For this review, take the finished solid that the model builds, in its own axes (mm). Round coordinates to 2 decimals unless told otherwise and drop trailing zeros. Loops run counter-clockwise (first coordinate to the right, second up) from the corner with the lowest first, then second, coordinate; pieces in that order, holes last.
1. Clearance check with flat-ended pins moving along their axes: pin 1 Ø10 at (x, y) = (-1.5, 80.5) entering from -Z; pin 2 Ø5.5 at (x, z) = (53.34, -76.18) entering from -Y; pin 3 Ø6.5 at (x, z) = (-92, 17) entering from -Y; pin 4 Ø8 at (y, z) = (87.5, 65.5) entering from -X. State where each tip first meets the part, or that it passes through.
2. To check wall thickness, follow line 1 along Z through (x, y) = (-49.5, 16); line 2 along Z through (x, y) = (29, 10); line 3 along Z through (x, y) = (0, 11). State the ranges of each line that lie inside material, in increasing order.
3. Draft analysis for pull direction Z (two halves, no side actions). For faces 1 (the flat face through (92, 13.7, -16)), 2 (the flat face through (-1, 0, -1)), 3 (the flat face through (86.75, 5.18, -33.3)), state which applies: released by +Z, released by -Z, zero draft, split by the parting line, or undercut.
4. Consider section A-A on x = 0. State the section outline as (y, z) points, then the cut area to 3 significant figures.
5. Consider section D-D on y = 52. State the section outline as (x, z) points.
6. Consider section B-B on y = 8. State the section outline as (x, z) points.
7. Consider section C-C on z = 44.5. State the section outline as (x, y) points.
Autodesk Fusion 360 part; units mm, degrees
sketch "Sketch1" plane through (0, 0, 0) normal (0, 0, 1) x (1, 0, 0)
  line L0 (0, 0) -> (102, 0)
  line L1 (0, 0) -> (0, 102)
  arc A0 (102, 0) -> (0, 102) centre (0, 0) ccw
  dimension "d1" = 204
revolve "Revolve1" add sketch "Sketch1" angle 360 about axis through (0, 0, 0) along (0, 1, 0)
sketch "Sketch2" plane through (0, 0, 0) normal (0, -1, 0) x (1, 0, 0)
  circle A0 centre (0, 0) radius 102
  line L0 (0, 0) -> (0, -0.5) construction
  line L1 (0, -0.5) -> (-40.4969, -0.5) construction
  line L2 (-40.4969, -0.5) -> (40.4969, -0.5)
  arc A1 (40.4969, -0.5) -> (-40.4969, -0.5) centre (0, 0) ccw
  dimension "d3" = 81
  dimension "d4" = 0.5
extrude "Extrude1" cut sketch "Sketch2" against normal blind 10.5 contours L2 A1
sketch "Sketch3" plane through (0, 0, 0) normal (0, -1, 0) x (1, 0, 0)
  line L0 (40.4969, -0.5) -> (-40.4969, -0.5)
  arc A0 (40.4969, -0.5) -> (-40.4969, -0.5) centre (0, 0) ccw
  circle A1 centre (0, 0) radius 102
sketch "Sketch4" plane through (0, 0, 0) normal (0, -1, 0) x (1, 0, 0)
  line L0 (0, 0) -> (0, -64) construction
  line L1 (40, -64) -> (40, -63)
  line L2 (40, -46.5) -> (-40, -81.5) construction
  line L3 (-40, -46.5) -> (0, -64) construction
  line L4 (0, -64) -> (0, -63)
  line L5 (0, -63) -> (-61.0824, -63)
  line L6 (0, -63) -> (61.0824, -63)
  line L7 (-40, -63) -> (-40, -64)
  arc A0 (-36.3095, -79.8854) -> (-32.524, -81.5) centre (0, 0) ccw
  line L8 (31.4468, 81.9217) -> (35.2097, 91.7243)
  line L9 (0, 0) -> (98.25, 0) construction
  line L10 (-31.4468, 81.9217) -> (-35.2097, 91.7243)
  line L11 (0, 0) -> (98.25, 0) construction
  line L12 (81.9217, 31.4468) -> (91.7243, 35.2097)
  line L13 (0, 0) -> (98.25, 0) construction
  line L14 (81.9217, -31.4468) -> (91.7243, -35.2097)
  line L15 (0, 0) -> (98.25, 0) construction
  line L16 (0, 114.2451) -> (0, -120) construction
  line L17 (-81.9217, 31.4468) -> (-91.7243, 35.2097)
  line L18 (-81.9217, -31.4468) -> (-91.7243, -35.2097)
  arc A1 (-81.9217, 31.4468) -> (-81.9217, -31.4468) centre (0, 0) ccw
  arc A2 (81.9217, -31.4468) -> (81.9217, 31.4468) centre (0, 0) ccw
  arc A3 (31.4468, 81.9217) -> (-31.4468, 81.9217) centre (0, 0) ccw
  arc A4 (35.2097, 91.7243) -> (-35.2097, 91.7243) centre (0, 0) ccw
  line L19 (-61.0824, -63) -> (-75.3927, -63)
  line L20 (61.0824, -63) -> (75.3927, -63)
  arc A5 (-91.7243, 35.2097) -> (-91.7243, -35.2097) centre (0, 0) ccw
  arc A6 (-75.3927, -63) -> (75.3927, -63) centre (0, 0) ccw
  arc A7 (91.7243, -35.2097) -> (91.7243, 35.2097) centre (0, 0) ccw
  point P0 (0, -64)
  dimension "d9" = 196.5
  dimension "d10" = 175.5
  dimension "d11" = 64
  dimension "d13" = 35
  dimension "d14" = 1
  dimension "d15" = 69
  dimension "d16" = 111
  dimension "d17" = 21
  dimension "d18" = 21
extrude "Extrude2" cut sketch "Sketch4" against normal blind 10.5
sketch "Sketch5" plane through (0, 0, 0) normal (0, -1, 0) x (1, 0, 0)
  circle A0 centre (0, 0) radius 93 construction
  line L0 (0, 0) -> (-16.1493, 91.5871) construction
  line L1 (0, 0) -> (93, 0) construction
  line L2 (0, 0) -> (16.1493, 91.5871) construction
  line L3 (0, 0) -> (93, 0) construction
  line L4 (0, 0) -> (-91.5871, 16.1493) construction
  line L5 (0, 0) -> (93, 0) construction
  line L6 (0, 0) -> (-91.5871, -16.1493) construction
  line L7 (0, 0) -> (93, 0) construction
  line L8 (0, 0) -> (91.5871, 16.1493) construction
  line L9 (0, 0) -> (93, 0) construction
  line L10 (0, 0) -> (91.5871, -16.1493) construction
  line L11 (0, 0) -> (93, 0) construction
  line L12 (0, 0) -> (0, -93) construction
  line L13 (0, 0) -> (-53.3426, -76.1811) construction
  line L14 (0, 0) -> (93, 0) construction
  line L15 (0, 0) -> (53.3426, -76.1811) construction
  circle A1 centre (0, 0) radius 20 construction
  line L16 (0, 0) -> (0, 20) construction
  circle A2 centre (-16.1493, 91.5871) radius 3
  circle A3 centre (16.1493, 91.5871) radius 3
  line L17 (0, 130) -> (0, -112.7435) construction
  circle A4 centre (-91.5871, 16.1493) radius 3
  circle A5 centre (-91.5871, -16.1493) radius 3
  circle A6 centre (-53.3426, -76.1811) radius 3
  circle A7 centre (91.5871, 16.1493) radius 3
  circle A8 centre (91.5871, -16.1493) radius 3
  circle A9 centre (53.3426, -76.1811) radius 3
  circle A10 centre (0, 20) radius 3
  circle A11 centre (0, -93) radius 3
  dimension "d21" = 186
  dimension "d22" = 100
  dimension "d23" = 80
  dimension "d24" = 170
  dimension "d25" = 170
  dimension "d26" = 10
  dimension "d27" = 10
  dimension "d28" = 125
  dimension "d29" = 40
  dimension "d30" = 6
  dimension "d31" = 6
  dimension "d32" = 6
  dimension "d33" = 6
  dimension "d34" = 6
  dimension "d35" = 6
  dimension "d36" = 6
extrude "Extrude3" cut sketch "Sketch5" against normal blind 13.7
Resolved:
1. pin 1: stops at z = -68.57
1. pin 2: stops at y = 13.7
1. pin 3: stops at y = 10.5
1. pin 4: passes through
2. line 1: z = -87.74 to 87.74
2. line 2: z = -97.28 to -93.87, -63 to -0.5, 28.27 to 82.82, 93.87 to 97.28
2. line 3: z = -101.41 to -96, -90 to 17, 23 to 101.41
3. face 1: undercut
3. face 2: zero draft
3. face 3: undercut
4. outline: (0, -102) arc R102 ccw to (0, 102) - (0, 98.25) - (10.5, 98.25) - (10.5, 87.75) - (0, 87.75) - (0, 40.5) - (10.5, 40.5) - (10.5, 23) - (13.7, 23) - (13.7, 17) - (10.5, 17) - (10.5, -0.5) - (0, -0.5) - (0, -63) - (10.5, -63) - (10.5, -90) - (13.7, -90) - (13.7, -96) - (10.5, -96) - (10.5, -98.25) - (0, -98.25) - close
4. area: 15,400 mm2
5. outline: circle Ø175.5 at (0, 0)
6. outline: circle Ø203.37 at (0, 0); hole (-91.72, -35.21) - (-81.92, -31.45) arc R87.75 cw to (-81.92, 31.45) - (-91.72, 35.21) arc R98.25 ccw to start; hole (-75.39, -63) arc R98.25 ccw to (75.39, -63) - close; hole (-40.5, -0.5) - (40.5, -0.5) arc R40.5 ccw (long way) to start; hole (-35.21, 91.72) - (-31.45, 81.92) arc R87.75 cw to (31.45, 81.92) - (35.21, 91.72) arc R98.25 ccw to start; hole (81.92, -31.45) - (91.72, -35.21) arc R98.25 ccw to (91.72, 35.21) - (81.92, 31.45) arc R87.75 cw to start
7. outline: (-91.78, 0) - (91.78, 0) arc R91.78 ccw to start
